Part model, mm, in its own coordinate system. A direction names the side the tool comes from. Give positions to 0.01 mm unless a question says otherwise; leave off trailing zeros. Order: outer loops, then holes, each group sorted by start corner. A loop starts at its lowest first (then second) coordinate and runs counter-clockwise, first axis right, second up. Notation, with made-up numbers: M 74,10 L 108,10 A16 cw 108,23 Z; hole C 27.5,35 d11. An arc over 180 degrees is marked long. Return JSON: item names as keys, results as strings.
from build123d import *

# Parameters (mm, degrees)
BOSS_EXTRUDE1_DEPTH = 40
BOSS_EXTRUDE2_DEPTH = 3
BOSS_EXTRUDE3_START = 25
BOSS_EXTRUDE3_DEPTH = 25
BOSS_EXTRUDE4_START = -12
BOSS_EXTRUDE4_DEPTH = 3


with BuildPart() as part:
    # Sketch1 → Boss-Extrude1 (new body)
    with BuildSketch(Plane.XY):
        with BuildLine():
            Line((-2.25, 5.25), (2.25, 5.25))
            ThreePointArc((2.25, 5.25), (4.371320344, 4.371320344), (5.25, 2.25))
            Line((5.25, 2.25), (5.25, -2.25))
            ThreePointArc((5.25, -2.25), (4.371320344, -4.371320344), (2.25, -5.25))
            Line((2.25, -5.25), (-2.25, -5.25))
            ThreePointArc((-2.25, -5.25), (-4.371320344, -4.371320344), (-5.25, -2.25))
            Line((-5.25, -2.25), (-5.25, 2.25))
            ThreePointArc((-5.25, 2.25), (-4.371320344, 4.371320344), (-2.25, 5.25))
        make_face()
    extrude(amount=BOSS_EXTRUDE1_DEPTH)

    # Sketch2 → Boss-Extrude2 (add, symmetric)
    with BuildSketch(Plane.XY):
        with BuildLine():
            Line((8.999999945, -3.000810302), (8.999999945, 2.999189698))
            ThreePointArc((8.999999945, 2.999189698), (8.121463527, 5.120366794), (6.000405096, 5.999189671))
            Line((6.000405096, 5.999189671), (-5.999594794, 6.000810275))
            ThreePointArc((-5.999594794, 6.000810275), (-8.121177041, 5.122273883), (-8.999999945, 3.000810302))
            Line((-8.999999945, 3.000810302), (-8.999999945, -2.999189698))
            ThreePointArc((-8.999999945, -2.999189698), (-8.121463527, -5.120366794), (-6.000405096, -5.999189671))
            Line((-6.000405096, -5.999189671), (5.999594794, -6.000810275))
            ThreePointArc((5.999594794, -6.000810275), (8.121177041, -5.122273883), (8.999999945, -3.000810302))
        make_face()
    extrude(amount=BOSS_EXTRUDE2_DEPTH, both=True)

    # Sketch3 → Boss-Extrude3 (add)
    with BuildSketch(Plane.XY.offset(3).offset(BOSS_EXTRUDE3_START)):
        with BuildLine():
            Line((0.000405151, 5.25), (-5.999999945, 5.25))
            ThreePointArc((-5.999999945, 5.25), (-7.590417233, 4.59122759), (-8.249189643, 3.000810302))
            Line((-8.249189643, 3.000810302), (-8.249189643, -2.999189698))
            ThreePointArc((-8.249189643, -2.999189698), (-7.590631979, -4.58939221), (-6.000607381, -5.248379314))
            Line((-6.000607381, -5.248379314), (0.000405151, -5.25))
            Line((0.000405151, -5.25), (0.000405151, -6.000000082))
            Line((0.000405151, -6.000000082), (-6.000405096, -5.999189671))
            ThreePointArc((-6.000405096, -5.999189671), (-8.121463527, -5.120366794), (-8.999999945, -2.999189698))
            Line((-8.999999945, -2.999189698), (-8.999999945, 3.000810302))
            ThreePointArc((-8.999999945, 3.000810302), (-8.121177041, 5.122273883), (-5.999594794, 6.000810275))
            Line((-5.999594794, 6.000810275), (0.000405151, 5.999999973))
            Line((0.000405151, 5.999999973), (0.000405151, 5.25))
        make_face()
    extrude(amount=-BOSS_EXTRUDE3_DEPTH)

    # Sketch5 → Boss-Extrude4 (add)
    with BuildSketch(Plane.XY.offset(40).offset(BOSS_EXTRUDE4_START)):
        with BuildLine():
            Line((0.000405151, -6.000000082), (5.999594794, -6.000810275))
            ThreePointArc((5.999594794, -6.000810275), (8.121177041, -5.122273883), (8.999999945, -3.000810302))
            Line((8.999999945, -3.000810302), (8.999999945, 2.999189698))
            ThreePointArc((8.999999945, 2.999189698), (8.121463527, 5.120366794), (6.000405096, 5.999189671))
            Line((6.000405096, 5.999189671), (0.000405151, 5.999999973))
            Line((0.000405151, 5.999999973), (-5.999594794, 6.000810275))
            ThreePointArc((-5.999594794, 6.000810275), (-8.121177041, 5.122273883), (-8.999999945, 3.000810302))
            Line((-8.999999945, 3.000810302), (-8.999999945, -2.999189698))
            ThreePointArc((-8.999999945, -2.999189698), (-8.121463527, -5.120366794), (-6.000405096, -5.999189671))
            Line((-6.000405096, -5.999189671), (0.000405151, -6.000000082))
        make_face()
    extrude(amount=-BOSS_EXTRUDE4_DEPTH)


solid = part.part
Q1. Pin check, flat tips, straight feed: pin 1 (2 mm diameter, centred on y = 4.5, z = 17, fed in from -X); pin 2 (9.5 mm diameter, centred on x = 2, z = 9, fed in from +Y); pin 3 (2 mm diameter, centred on y = -1, z = 32, fed in from +X); pin 4 (5 mm diameter, centred on x = 0, z = 33.5, fed in from -Y). Stop position of each tip, or through.
Established:
{"pin 1": "stops at x = -8.96", "pin 2": "stops at y = 6", "pin 3": "stops at x = 5.25", "pin 4": "stops at y = -5.25"}
Q2. Band-saw the part on A-A (y = 1.5). Give the cut face in (x, z), then the cut area to 3 significant figures.
Established:
{"outline": "M -9,-3 L 9,-3 L 9,3 L 5.25,3 L 5.25,25 L 9,25 L 9,28 L 5.25,28 L 5.25,40 L -5.25,40 L -5.25,28 L -9,28 Z; hole M -8.25,3 L -5.25,3 L -5.25,25 L -8.25,25 Z", "area": "536 mm²"}
Q3. 3-axis set-ups, long thin cutter, end or side, ignore diameter. For faces 1 (the cylindrical face through (4.35, 4.39, 13.85)), 2 (the flat face through (-5.25, 0, 34)), 3 (the flat face through (5.25, 0, 34)), 4 (the flat face through (-8.249, 0, 14)), 5 (the flat face through (0, -5.25, 34)): which of +Z, -Z, +X, -X, +Y, -Y reach the whole face in a straight line?
Established:
{"face 1": "+X, +Y", "face 2": "+Z, -X, +Y, -Y", "face 3": "+Z, +X, +Y, -Y", "face 4": "none", "face 5": "+Z, +X, -X, -Y"}
Q4. Band-saw the part on C-C (x = 4.75). Give the cut face in (y, z).
Established:
{"outline": "M -6,-3 L 6,-3 L 6,3 L 3.91,3 L 3.91,25 L 6,25 L 6,28 L 3.91,28 L 3.91,40 L -3.91,40 L -3.91,28 L -6,28 L -6,25 L -3.91,25 L -3.91,3 L -6,3 Z"}
Q5. Two-plate mould, pull along X, no slides. Class faces 6 (the cylindrical face through (-4.39, 4.35, 13.85)), 7 (the cylindrical face through (4.39, -4.35, 13.85)), 8 (the flat face through (0, 0, 40)): +X half, -X half, draft (parallel to the pull), parting line (faces both ways), or undercut.
Established:
{"face 6": "undercut", "face 7": "+X half", "face 8": "draft"}
Q6. Band-saw the part on B-B (z = 11). Give the cut face in (x, y), then the cut area to 3 significant figures.
Established:
{"outline": "M -9,-3 A3 ccw -6,-6 L 0,-6 L 0,-5.25 L 2.25,-5.25 A3 ccw 5.25,-2.25 L 5.25,2.25 A3 ccw 2.25,5.25 L 0,5.25 L 0,6 L -6,6 A3 ccw -9,3 Z; hole M -8.25,-3 A2.25 ccw -6,-5.25 L -2.31,-5.25 A3 cw -5.25,-2.25 L -5.25,2.25 A3 cw -2.25,5.25 L -6,5.25 A2.25 ccw -8.25,3 Z", "area": "122 mm²"}
Q7. Band-saw the part on D-D (z = 31.5). Give the cut face in (x, y), then the cut area to 3 significant figures.
Established:
{"outline": "M -5.25,-2.25 A3 ccw -2.25,-5.25 L 2.25,-5.25 A3 ccw 5.25,-2.25 L 5.25,2.25 A3 ccw 2.25,5.25 L -2.25,5.25 A3 ccw -5.25,2.25 Z", "area": "103 mm²"}
Q8. Probe line 1 along Z through (x, y) = (6.5, 0.5); line 2 along X through (y, z) = (1.5, 15); line 3 along Y through (x, z) = (-4.25, 19.5). List the from-to ranges inside material, lowest first.
Established:
{"line 1": "z = -3 to 3, 25 to 28", "line 2": "x = -9 to -8.25, -5.25 to 5.25", "line 3": "y = -6 to -5.25, -4.49 to 4.49, 5.25 to 6"}
